Answer from the drawing. Dimensions are ordinates in mm from the lowest x, y and z of the part. A direction names the side the tool comes from. Coordinates: 2 decimals unless noted, no trailing zeros. Write each loop counter-clockwise with the first axis right and the second up, starting at its lowest first coordinate (ties: lowest second). Pieces come first, ordered by that corner, then holes. Notation, with made-up numbers: (62, 29) - (111, 29) arc R20 ccw to (111, 58) - close; hole circle Ø4 at (-17, -1). An arc over 180 degrees is marked (long way). Return JSON: item names as keys, results as strings.
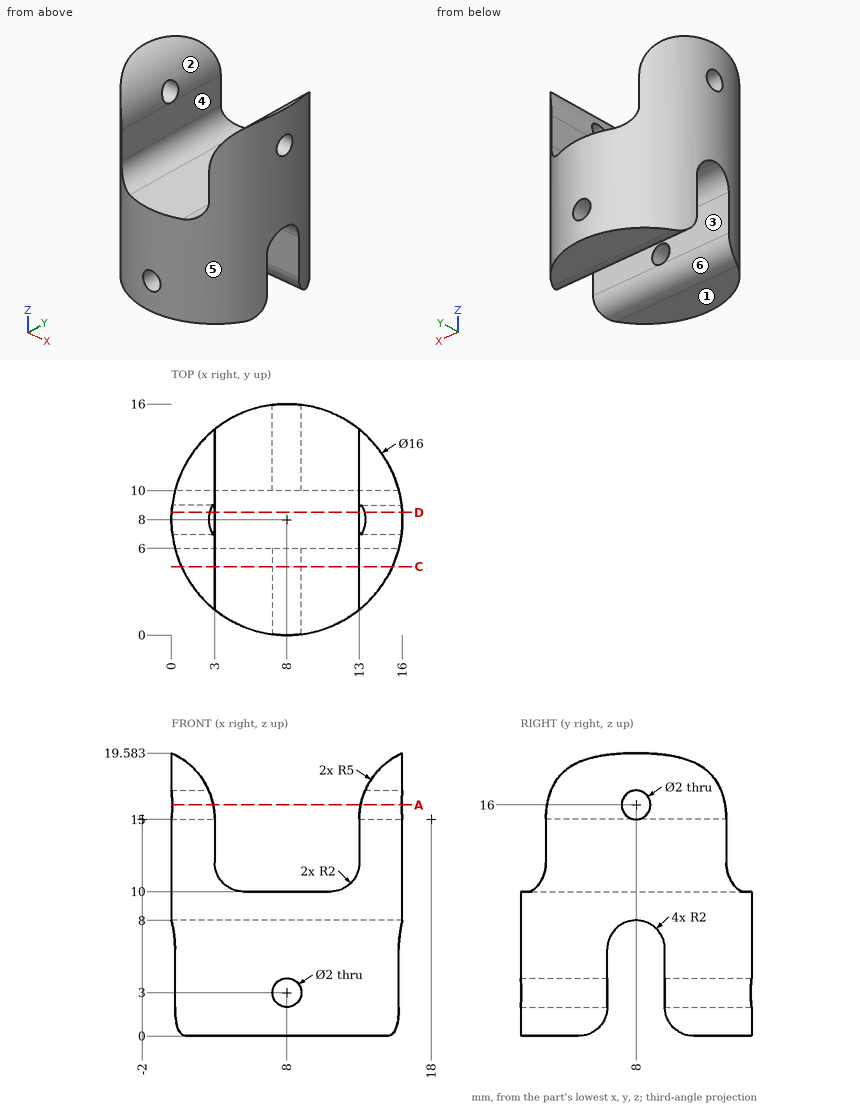
(1) Straight lines are drawn through the part: line 1 (Y direction, x = 11, z = 9.5); line 2 (Y direction, x = 9.5, z = 6.25) (1 decimal); line 3 (Y direction, x = 8.5, z = 1.25) (1 decimal). For each, find the intervals that lie inside material, in ascending order. Write a range as from..to.
Answer:
{"line 1": "0.58..15.42", "line 2": "0.1..6, 10..15.9", "line 3": "0..5.9, 10.1..16"}
(2) A cutting plane is placed at D-D (y = 8.5). Determine the outline of the cut face in (x, z).
Answer:
{"outline": "(0.02, 7.94) - (15.98, 7.94) - (15.98, 15.13) - (13, 15.13) arc R5 ccw to (13, 15.03) - (13, 12) arc R2 cw to (11, 10) - (5, 10) arc R2 cw to (3, 12) - (3, 15.03) arc R5 ccw to (3, 15.13) - (0.02, 15.13) - close; (0.02, 16.87) - (2.64, 16.87) arc R5 ccw to (0.02, 19.58) - close; (13.36, 16.87) - (15.98, 16.87) - (15.98, 19.58) arc R5 ccw to start"}
(3) Determine the mould class of the marked faces 4, 5 and 6 for opening direction Y: +Y half, -Y half, draft (parallel to the pull), parting line (faces both ways), or undercut.
Answer:
{"face 4": "draft", "face 5": "parting line", "face 6": "undercut"}
(4) A cutting plane is placed at C-C (y = 4.75). Determine the outline of the cut face in (x, z) (1 decimal).
Answer:
{"outline": "(0.7, 0.1) - (15.3, 0.1) - (15.3, 19.2) arc R5 ccw to (13, 15) - (13, 12) arc R2 cw to (11, 10) - (5, 10) arc R2 cw to (3, 12) - (3, 15) arc R5 ccw to (0.7, 19.2) - close; hole circle Ø2 at (8, 3)"}
(5) Which of the six approach directions +Z, -Z, +X, -X, +Y, -Y give full straight-line access (tool end or side, diameter ignored) to the marked faces 1, 2 and 3?
Answer:
{"face 1": "-Z, +X, -X, +Y, -Y", "face 2": "+Z, +Y, -Y", "face 3": "-Z, +X, -X"}
(6) Flat-ended cylindrical pins translate along their axes: P1, Ø1, axis at y = 13.5, z = 15, coming from the +X side (1 decimal); P2, Ø2, axis at x = 13.5, z = 12, coming from the +Y side; P3, Ø6.5, axis at x = 9, y = 11.5, coming from the +Z side; P4, Ø4, axis at x = 5.5, z = 16, coming from the +Y side. Find the tip coordinate at first contact, or state that the pin passes through.
Answer:
{"P1": "x = 14.2", "P2": "y = 14.36", "P3": "z = 10.44", "P4": "through"}
(7) A cutting plane is placed at A-A (z = 16). Determine the outline of the cut face in (x, y).
Answer:
{"outline": "(0.06, 7) arc R8 ccw to (2.9, 1.84) - (2.9, 7) - close; (0.06, 9) - (2.9, 9) - (2.9, 14.16) arc R8 ccw to start; (13.1, 1.84) arc R8 ccw to (15.94, 7) - (13.1, 7) - close; (13.1, 9) - (15.94, 9) arc R8 ccw to (13.1, 14.16) - close"}
